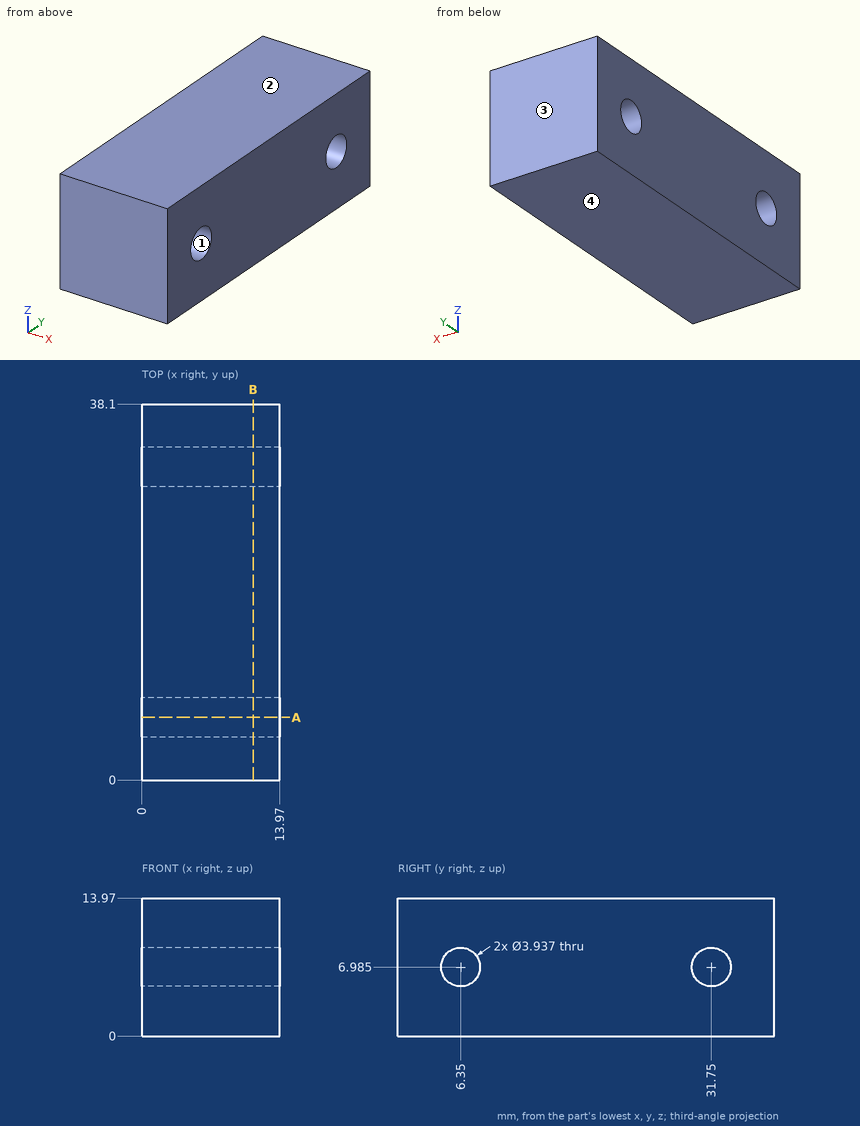
Design review of the part shown in the three views and the two pictorial views. Dimensions are in mm from the part's minimum x, y and z. Give positions to 0.01 mm unless a question says otherwise; leave off trailing zeros. Loops run counter-clockwise (first coordinate to the right, second up) from the corner with the lowest first, then second, coordinate; pieces in that order, holes last. Notation, with made-up numbers: (2.25, 25) -> (36.25, 25) arc R17 cw to (36.25, 58) -> close; hole circle Ø6 at (10, 78.5). An arc over 180 degrees is marked (long way). Put each result on its own line as item: value. Start each with the question number.
1. Wall thickness on probe 1 along Z at (x, y) = (9.5, 31.75); probe 2 along Y at (x, z) = (6.25, 8.75); probe 3 along Y at (x, z) = (3.25, 5.25): over which ranges is each line inside the solid? List them lowest first.
2. Clearance check with a flat-ended pin moving along its axis: P1, Ø3.5, axis at y = 31.75, z = 6.985, coming from the +X side (3 decimals). State where the tip first meets the part, or that it passes through.
3. We need section A-A on y = 6.35. State the section outline as (x, z) points.
4. We need section B-B on x = 11.25. State how many separate pieces and enclosed holes the cut face has, then the cut area to 3 significant figures.
5. Mouldability with a two-part tool opening along Z and no side actions: class the marked faces 1, 2, 3 and 4 as released by +Z, released by -Z, zero draft, split by the parting line, or undercut.
Determined:
1. probe 1: 0 to 5.02, 8.95 to 13.97
1. probe 2: 0 to 5.48, 7.22 to 30.88, 32.62 to 38.1
1. probe 3: 0 to 5.42, 7.28 to 30.82, 32.68 to 38.1
2. P1: through
3. outline: (0, 0) -> (13.97, 0) -> (13.97, 5.02) -> (0, 5.02) -> close; (0, 8.95) -> (13.97, 8.95) -> (13.97, 13.97) -> (0, 13.97) -> close
4. separate pieces: 1
4. enclosed holes: 2
4. area: 508 mm^2
5. face 1: undercut
5. face 2: released by +Z
5. face 3: zero draft
5. face 4: released by -Z
